```python
from build123d import *

# Parameters (mm, degrees)
EXTRUDE_1_DEPTH = 1.6
SKETCH_2_W      = 4.925580802
SKETCH_2_H      = 4.825372048
EXTRUDE_2_DEPTH = 1.6


with BuildPart() as part:
    # 草图1 → 凸台-拉伸1 (new body)
    with BuildSketch(Plane.XY):
        with BuildLine():
            Line((-5.408326913, 1), (-7.608326913, 1))
            Line((-7.608326913, 1), (-7.608326913, -1))
            Line((-7.608326913, -1), (-5.408326913, -1))
            ThreePointArc((-5.408326913, -1), (5.5, 0), (-5.408326913, 1))
        make_face()
    extrude(amount=EXTRUDE_1_DEPTH)

    # 草图2 → 凸台-拉伸2 (add)
    with BuildSketch(Plane.XY.offset(1.6)):
        Rectangle(SKETCH_2_W, SKETCH_2_H)
    extrude(amount=EXTRUDE_2_DEPTH)


solid = part.part
```
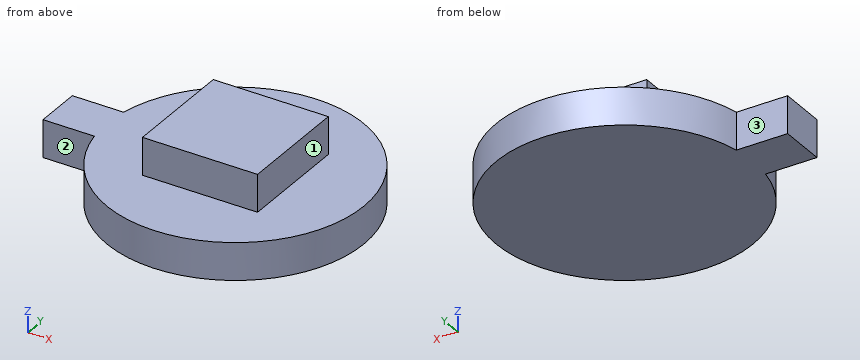
Can you work these out from the model? Positions are in its coordinate system, mm. Face numbers are marked on the shaded views. A direction names the side the tool comes from. Give positions to 0.01 mm unless a question says otherwise; leave off trailing zeros. Loops run counter-clockwise (first coordinate to the right, second up) from the corner with the lowest first, then second, coordinate; pieces in that order, holes last. Notation, with made-up numbers: M -33.75,84.5 L -13.75,84.5 A38 cw -13.75,123.5 Z; hole C -12.5,-37 d4. An arc over 180 degrees is marked long. Answer in a Markdown table with one row per item.
1. Suppose I cut it at D-D on x = 3.5. Write out the boundary of the cut face in (y, z).
Taken from the geometry:
| item | result |
|---|---|
| outline | M -4.24,0 L 4.24,0 L 4.24,1.6 L -4.24,1.6 Z |
2. If I drill on line 1 along X through (y, z) = (0.25, 2.3); line 2 along Z through (x, y) = (2.5, 0.5); line 3 along Y through (x, z) = (-1.75, 2.6), over which ranges is the centre line in solid material (lowest first)?
Taken from the geometry:
| item | result |
|---|---|
| line 1 | x = -2.46 to 2.46 |
| line 2 | z = 0 to 1.6 |
| line 3 | y = -2.41 to 2.41 |
3. For pin 1 Ø1.3 at (x, z) = (-7, 0.5) entering from -Y; pin 2 Ø0.5 at (x, z) = (0.5, 2) entering from +Y; pin 3 Ø0.5 at (x, z) = (0.5, 2) entering from -Y, each with a flat end and sliding along its axis, tell me the tip position at first contact or that it passes through.
Taken from the geometry:
| item | result |
|---|---|
| pin 1 | stops at y = -1 |
| pin 2 | stops at y = 2.41 |
| pin 3 | stops at y = -2.41 |
4. Which directions (+Z, -Z, +X, -X, +Y, -Y) give clear straight access to the entire face, cutting with the end or side of a thin tool? Please do the marked faces 1, 2 and 3.
Taken from the geometry:
| item | result |
|---|---|
| face 1 | +Z, +X, +Y, -Y |
| face 2 | +Z, -Z, -X, -Y |
| face 3 | +Z, -Z, -X, +Y |
5. Suppose I cut it at A-A on y = 0. Write out the boundary of the cut face in (x, z), plus the area to 3 significant figures.
Taken from the geometry:
| item | result |
|---|---|
| outline | M -7.61,0 L 5.5,0 L 5.5,1.6 L 2.46,1.6 L 2.46,3.2 L -2.46,3.2 L -2.46,1.6 L -7.61,1.6 Z |
| area | 28.9 mm² |
6. Suppose I cut it at B-B on x = 0. Write out the boundary of the cut face in (y, z), plus the area to 3 significant figures.
Taken from the geometry:
| item | result |
|---|---|
| outline | M -5.5,0 L 5.5,0 L 5.5,1.6 L 2.41,1.6 L 2.41,3.2 L -2.41,3.2 L -2.41,1.6 L -5.5,1.6 Z |
| area | 25.3 mm² |
7. Suppose I cut it at C-C on z = 2.45. Write out the boundary of the cut face in (x, y), plus the area to 3 significant figures.
Taken from the geometry:
| item | result |
|---|---|
| outline | M -2.46,-2.41 L 2.46,-2.41 L 2.46,2.41 L -2.46,2.41 Z |
| area | 23.8 mm² |
